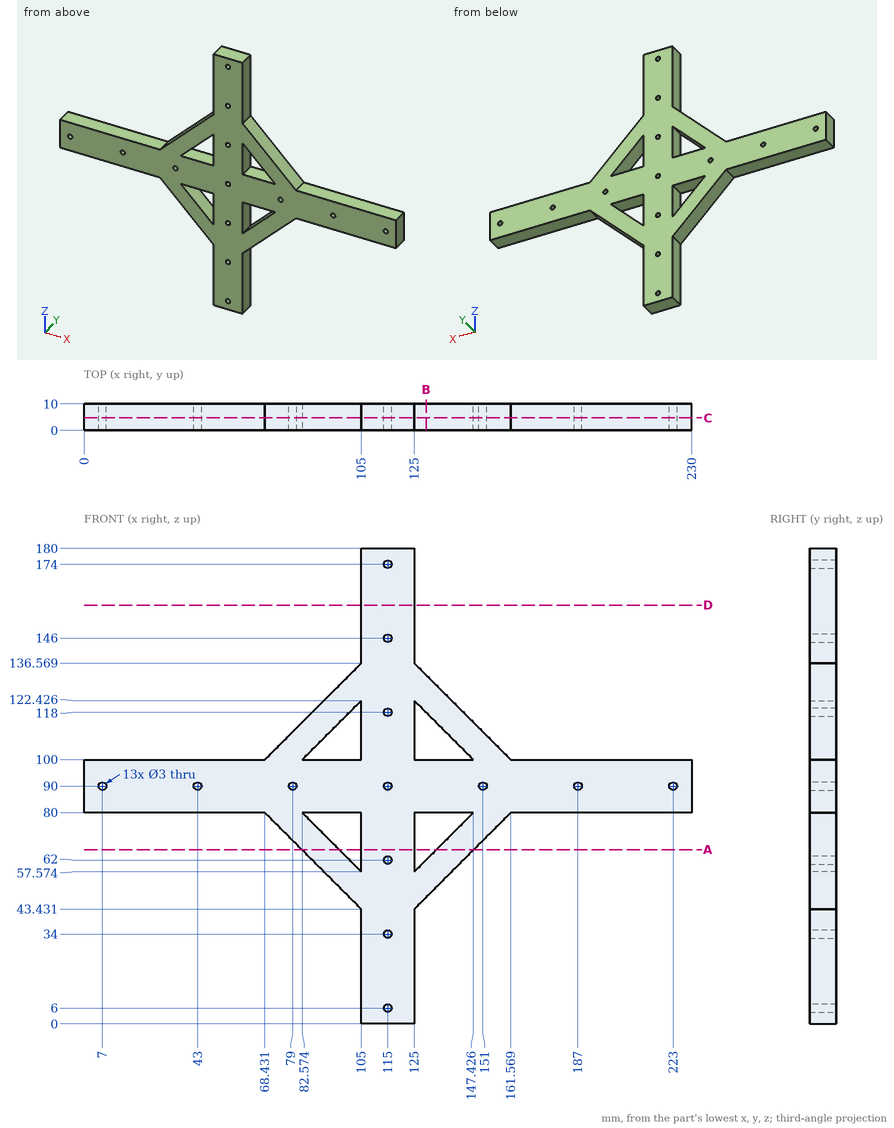
Drawing for the job (mm, zero at the part's lowest x, y, z). Give positions to 0.01 mm unless a question says otherwise; leave off trailing zeros. Order: outer loops, then holes, each group sorted by start corner. A loop starts at its lowest first (then second) coordinate and runs counter-clockwise, first axis right, second up. Notation, with made-up numbers: M 72.5,6 L 128.5,6 A16 ccw 128.5,28 Z; hole C 39,27.25 d2. An arc over 180 degrees is marked long. Write item = value, one per line. Start each with the question number.
(1) Probe L1, parallel to Z at x = 223, y = 7; L2, parallel to X at y = 7, z = 62 (1 decimal); L3, parallel to Z at x = 136.5, y = 4.75 (1 decimal). List the from-to ranges inside material, lowest first. Write a range as [from, to].
(2) Pin check, flat tips, straight feed: pin 1 Ø4 at (x, z) = (151, 90) entering from +Y; pin 2 Ø4 at (y, z) = (4, 58) entering from -X; pin 3 Ø2 at (y, z) = (5.5, 59.5) entering from -X; pin 4 Ø2 at (y, z) = (5.5, 65) entering from +X. Stop position of each tip, or through.
(3) Slice it at B-B on x = 129.5. Write the cut outline in (y, z).
(4) Slice it at D-D on z = 158.5. Write the cut outline in (x, y).
(5) Slice it at A-A on z = 66. Write the cut outline in (x, y), plus the area to 3 significant figures.
(6) Slice it at C-C on y = 4.75. State how many separate pieces and enclosed holes the cut face has, plus the area to 3 significant figures.
Responses:
q1.L1 = [80, 88.5], [91.5, 100]
q1.L2 = [86.4, 100.6], [105, 113.5], [116.5, 125], [129.4, 143.6]
q1.L3 = [54.9, 69.1], [80, 100], [110.9, 125.1]
q2.pin_1 = 10
q2.pin_2 = 88.43
q2.pin_3 = 87.93
q2.pin_4 = 147.57
q3.outline = M 0,47.93 L 10,47.93 L 10,62.07 L 0,62.07 Z; M 0,80 L 10,80 L 10,100 L 0,100 Z; M 0,117.93 L 10,117.93 L 10,132.07 L 0,132.07 Z
q4.outline = M 105,0 L 125,0 L 125,10 L 105,10 Z
q5.outline = M 82.43,0 L 96.57,0 L 96.57,10 L 82.43,10 Z; M 105,0 L 125,0 L 125,10 L 105,10 Z; M 133.43,0 L 147.57,0 L 147.57,10 L 133.43,10 Z
q5.area = 483 mm2
q6.separate_pieces = 1
q6.enclosed_holes = 17
q6.area = 9,380 mm2
